Could you check a few things on this model? Use its own coordinates, in mm. A direction names the side the tool comes from. Round coordinates to 2 decimals unless told otherwise and drop trailing zeros. Order: outer loops, then holes, each group sorted by start corner. A loop starts at its lowest first (then second) coordinate and runs counter-clockwise, first axis right, second up. Notation, with made-up numbers: (12.25, 75.25) -> (38.25, 75.25) arc R21 ccw to (38.25, 104.25) -> close; hole circle Ø3 at (89.25, 16.25). An arc over 180 degrees is marked (long way). Put each result on its own line as item: value. Start each with the question number.
from build123d import *

# Parameters (mm, degrees)
SKETCH1_R          = 26
PLATE_DEPTH        = 8
SKETCH2_W          = 3.75
SKETCH2_H          = 28
DRIVE_LUG_DEPTH    = 8
SKETCH6_R          = 1
CUT_EXTRUDE5_DEPTH = 4.5


with BuildPart() as part:
    # Sketch1 → PLATE (new body)
    with BuildSketch(Plane.XY):
        Circle(SKETCH1_R)
    extrude(amount=PLATE_DEPTH)

    # Sketch2 → DRIVE_LUG (add)
    with BuildSketch(Plane.XY):
        with Locations((-11.125, 34)):
            Rectangle(SKETCH2_W, SKETCH2_H)
    extrude(amount=DRIVE_LUG_DEPTH)

    # Sketch6 → Cut-Extrude5 (cut)
    with BuildSketch(Plane(origin=(0, 0, 0), x_dir=(-1, 0, 0), z_dir=(0, 0, -1))):
        with Locations((11.25, 45.5)):
            Circle(SKETCH6_R)
    extrude(amount=-CUT_EXTRUDE5_DEPTH, mode=Mode.SUBTRACT)


solid = part.part
1. If we section it at C-C, the plane z = 6.5: Please give me the cut outline in (x, y).
2. I need wall thicknesses on L1, parallel to Y at x = -11.25, z = 1.7; L2, parallel to X at y = 35, z = 7.5; L3, parallel to Y at x = 6, z = 3.5. Which ranges of each line are inside material? Lowest first, please.
3. If we section it at B-B, the plane x = 0: Please give me the cut outline in (y, z), then the cut area to 3 significant figures.
4. If we section it at D-D, the plane x = -11.25: Please give me the cut outline in (y, z), then the cut area to 3 significant figures.
5. If we section it at A-A, the plane z = 1.5: Please give me the cut outline in (x, y).
6. For pin 1 Ø2.5 at (y, z) = (38.5, 3.5) entering from -X; pin 2 Ø1.8 at (x, y) = (-11.25, 45.5) entering from -Z; pin 3 Ø4 at (y, z) = (38.5, 1.5) entering from +X, each with a flat end and sliding along its axis, tell me the tip position at first contact or that it passes through.
7. Thinking about a two-plate mould opening in Y: for faces 4 (the face through (-11.12, 46.49, 2.22)), 5 (the face through (-9.25, 36, 4)), 6 (the face through (-11, 48, 4)), which applies, +Y half, -Y half, draft (parallel to the pull), parting line (faces both ways), or undercut?
8. Which directions (+Z, -Z, +X, -X, +Y, -Y) give clear straight access to the entire face, cutting with the end or side of a thin tool? Please do faces 1 (the face through (-13, 35, 4)), 2 (the face through (0, 3, 8)), 3 (the face through (-11, 46, 4.5)).
Results below:
1. outline: (-13, 22.52) arc R26 ccw (long way) to (-9.25, 24.3) -> (-9.25, 48) -> (-13, 48) -> close
2. L1: -23.44 to 44.5, 46.5 to 48
2. L2: -13 to -9.25
2. L3: -25.3 to 25.3
3. outline: (-26, 0) -> (26, 0) -> (26, 8) -> (-26, 8) -> close
3. area: 416 mm2
4. outline: (-23.44, 0) -> (44.5, 0) -> (44.5, 4.5) -> (46.5, 4.5) -> (46.5, 0) -> (48, 0) -> (48, 8) -> (-23.44, 8) -> close
4. area: 563 mm2
5. outline: (-13, 22.52) arc R26 ccw (long way) to (-9.25, 24.3) -> (-9.25, 48) -> (-13, 48) -> close; hole circle Ø2 at (-11.25, 45.5)
6. pin 1: x = -13
6. pin 2: z = 4.5
6. pin 3: x = -9.25
7. face 4: undercut
7. face 5: draft
7. face 6: +Y half
8. face 1: +Z, -Z, -X, +Y
8. face 2: +Z, +X, -X, +Y, -Y
8. face 3: -Z
